Geometry: final body of the model. Coordinates: model frame, mm. Face numbers are marked on the shaded views. Give positions to 0.01 mm unless a question says otherwise; leave off trailing zeros. Write each loop counter-clockwise with the first axis right and the second up, starting at its lowest first coordinate (ties: lowest second). Pieces come first, ordered by that corner, then holes. Notation, with made-up numbers: M 72.25,35 L 118.25,35 A19 ccw 118.25,56 Z; hole C 44,-37.5 d1. An arc over 180 degrees is marked long. Answer as a JSON object with one key per item and string values.
from build123d import *

# Parameters (mm, degrees)
SKETCH_1_W          = 875
SKETCH_1_H          = 900
EXTRUDE_1_DEPTH     = 1.5
SKETCH_2_W          = 875
SKETCH_2_H          = 900
SKETCH_2_W_2        = 872
SKETCH_2_H_2        = 897
EXTRUDE_2_DEPTH     = 15
SKETCH_3_W          = 875
SKETCH_3_H          = 900
SKETCH_3_W_2        = 845
SKETCH_3_H_2        = 880
EXTRUDE_3_DEPTH     = 1.5
SKETCH_6_R          = 3
CUT_EXTRUDE_1_DEPTH = 19
FILLET_1_R          = 1


with BuildPart() as part:
    # 草图1 → 凸台-拉伸1 (new body)
    with BuildSketch(Plane.XY):
        Rectangle(SKETCH_1_W, SKETCH_1_H)
    extrude(amount=EXTRUDE_1_DEPTH)

    # 草图2 → 凸台-拉伸2 (add)
    with BuildSketch(Plane(origin=(0, 0, 0), x_dir=(-1, 0, 0), z_dir=(0, 0, -1))):
        Rectangle(SKETCH_2_W, SKETCH_2_H)
        Rectangle(SKETCH_2_W_2, SKETCH_2_H_2, mode=Mode.SUBTRACT)
    extrude(amount=EXTRUDE_2_DEPTH)

    # 草图3 → 凸台-拉伸3 (add)
    with BuildSketch(Plane(origin=(0, 0, -15), x_dir=(-1, 0, 0), z_dir=(0, 0, -1))):
        Rectangle(SKETCH_3_W, SKETCH_3_H)
        Rectangle(SKETCH_3_W_2, SKETCH_3_H_2, mode=Mode.SUBTRACT)
    extrude(amount=EXTRUDE_3_DEPTH)

    # 草图6 → 切除-拉伸1 (cut, through all)
    with BuildSketch(Plane.XY.offset(1.5)):
        with Locations((-408.5, -421)):
            Circle(SKETCH_6_R)
        with Locations((408.5, -421)):
            Circle(SKETCH_6_R)
    extrude(amount=-CUT_EXTRUDE_1_DEPTH, mode=Mode.SUBTRACT)

    # 圆角1
    fillet_1_edges = [part.edges().sort_by_distance(p)[0] for p in [
        (437.5, 0, 1.5),
        (0, 450, 1.5),
        (-437.5, 0, -16.5),
        (0, 450, -16.5),
        (437.5, 0, -16.5),
        (0, -450, -16.5),
        (-437.5, 0, 1.5),
        (0, -450, 1.5),
        (-437.5, 450, -7.5),
        (437.5, 450, -7.5),
        (437.5, -450, -7.5),
        (-437.5, -450, -7.5),
    ]]
    fillet(fillet_1_edges, radius=FILLET_1_R)


solid = part.part
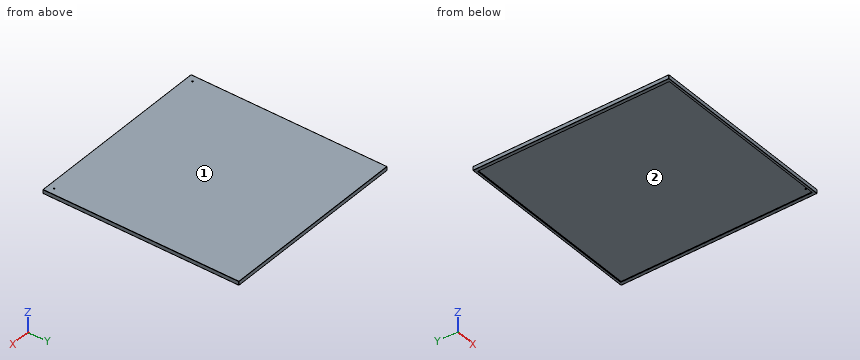
1) Cut plane C-C on z = -7.25. Return loops of the section in (x, y), and give its area (3 significant figures).
Geometry check:
{"outline": "M -437.5,-449 A1 ccw -436.5,-450 L 436.5,-450 A1 ccw 437.5,-449 L 437.5,449 A1 ccw 436.5,450 L -436.5,450 A1 ccw -437.5,449 Z; hole M -436,-448.5 L 436,-448.5 L 436,448.5 L -436,448.5 Z", "area": "5,320 mm2"}
2) Cut plane A-A on y = 204.5. Return loops of the section in (x, z).
Geometry check:
{"outline": "M -437.5,-15.5 A1 ccw -436.5,-16.5 L -422.5,-16.5 L -422.5,-15 L -436,-15 L -436,0 L 436,0 L 436,-15 L 422.5,-15 L 422.5,-16.5 L 436.5,-16.5 A1 ccw 437.5,-15.5 L 437.5,0.5 A1 ccw 436.5,1.5 L -436.5,1.5 A1 ccw -437.5,0.5 Z"}
3) Pull-direction query (Y, two-part tool) for the marked faces 1 and 2; classes: pulls with the +Y half, pulls with the -Y half, needs draft (parallel to the pull), parting line crosses it, or undercut.
Geometry check:
{"face 1": "needs draft", "face 2": "undercut"}
4) Cut plane B-B on x = 250.5. Return loops of the section in (y, z), and give its area (3 significant figures).
Geometry check:
{"outline": "M -450,-15.5 A1 ccw -449,-16.5 L -440,-16.5 L -440,-15 L -448.5,-15 L -448.5,0 L 448.5,0 L 448.5,-15 L 440,-15 L 440,-16.5 L 449,-16.5 A1 ccw 450,-15.5 L 450,0.5 A1 ccw 449,1.5 L -449,1.5 A1 ccw -450,0.5 Z", "area": "1,420 mm2"}
5) Contact query for flat-ended pins moving along their axis: P1, Ø12, axis at x = 236.5, y = -237.5, coming from the -Z side; P2, Ø3.5, axis at x = -408.5, y = -421, coming from the -Z side. Output: stop coordinate, or through.
Geometry check:
{"P1": "stops at z = 0", "P2": "passes through"}
6) Line query: line 1 (X direction, y = -421, z = 0.9); line 2 (X direction, y = -421, z = 1.1); line 3 (X direction, y = -119, z = -11). Output: solid intervals per line, ascending. Write a range as from..to.
Geometry check:
{"line 1": "x = -437.42..-411.5, -405.5..405.5, 411.5..437.42", "line 2": "x = -437.3..-411.5, -405.5..405.5, 411.5..437.3", "line 3": "x = -437.5..-436, 436..437.5"}
